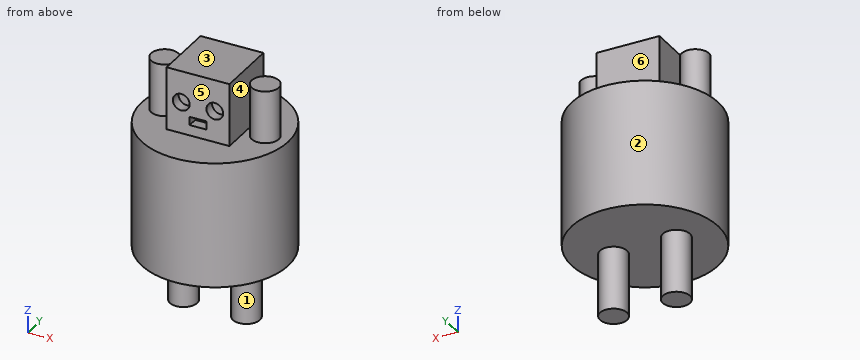
```python
from build123d import *

# Parameters (mm, degrees)
F0_W     = 30
F0_H     = 30
F1_DEPTH = 15
F2_R     = 35
F3_DEPTH = 60
F4_R     = 6.5
F5_DEPTH = 30
F6_R     = 4
F6_W     = 8
F6_H     = 4
F7_DEPTH = 5
F8_R     = 6.5
F9_DEPTH = 25


with BuildPart() as f1:
    # F0 (on Front) → F1 (new body, symmetric)
    with BuildSketch(Plane.XZ):
        with Locations((0, 40)):
            Rectangle(F0_W, F0_H)
    extrude(amount=F1_DEPTH, both=True)

    # F2 (on face) → F3 (join)
    with BuildSketch(Plane(origin=(0, 0, 25), x_dir=(1, 0, 0), z_dir=(0, 0, -1))):
        Circle(F2_R)
    extrude(amount=F3_DEPTH)

    # F4 (on face) → F5 (join)
    with BuildSketch(Plane(origin=(0, 0, -35), x_dir=(1, 0, 0), z_dir=(0, 0, -1))):
        with Locations((-15, 0)):
            Circle(F4_R)
        with Locations((15, 0)):
            Circle(F4_R)
    extrude(amount=F5_DEPTH)

    # F6 (on face) → F7 (cut)
    with BuildSketch(Plane.XZ.offset(15)):
        with Locations((-8, 40)):
            Circle(F6_R)
        with Locations((8, 40)):
            Circle(F6_R)
        with Locations((0, 32)):
            Rectangle(F6_W, F6_H)
    extrude(amount=-F7_DEPTH, mode=Mode.SUBTRACT)

    # F8 (on face) → F9 (join)
    with BuildSketch(Plane.XY.offset(25)):
        with Locations((-24, 0)):
            Circle(F8_R)
        with Locations((24, 0)):
            Circle(F8_R)
    extrude(amount=F9_DEPTH)


solid = f1.part
```
Check sheet for the modelled part. Datum: model origin and axes. Units: mm. Face numbers are marked on the shaded views. A direction names the side the tool comes from. Round coordinates to 2 decimals unless told otherwise and drop trailing zeros. Order: outer loops, then holes, each group sorted by start corner. A loop starts at its lowest first (then second) coordinate and runs counter-clockwise, first axis right, second up. Notation, with made-up numbers: (-38, -28) -> (-32, -28) arc R23 cw to (-32, -14) -> close; hole circle Ø10 at (45, -30.75). An arc over 180 degrees is marked (long way). One line per item, written item: value. Start each with the question number.
Q1. Cross-section at A-A (z = 40). Record the boundary of the cut face in (x, y), and give its area (3 significant figures).
Q2. Cross-section at B-B (x = 0). Record the boundary of the cut face in (y, z).
Q3. Gauge pin test, flat ends, axial feed: pin 1 Ø2 at (y, z) = (-13.5, 32) entering from -X; pin 2 Ø10.5 at (x, z) = (8, 40) entering from +Y; pin 3 Ø24 at (x, z) = (-3, 46.5) entering from -Y; pin 4 Ø21 at (x, y) = (9, -4.5) entering from -Z. Record the tip position at first contact, or that the pin passes through.
Q4. Set-up check for the marked faces 4, 5 and 6: record each of +Z, -Z, +X, -X, +Y, -Y from which the full face is reachable in a straight line by a thin tool's end or side.
Q5. Cross-section at C-C (z = -48). Record the boundary of the cut face in (x, y), and give its area (3 significant figures).
Q6. Mould release check, pull along X, two halves, no side actions. Record for the marked faces 1, 2 and 3: pulls with the +X half, pulls with the -X half, needs draft (parallel to the pull), parting line crosses it, or undercut.
Q7. Thickness scan on line 1 (Z direction, x = 8, y = -11.55); line 2 (X direction, y = 6, z = 25.5); line 3 (Z direction, x = 18, y = 20). Record the ranges inside material, lowest first.
Q8. Cross-section at D-D (y = 0). Record the boundary of the cut face in (x, z), and give its area (3 significant figures).
Completed:
1. outline: circle Ø13 at (-24, 0); (-15, -15) -> (-12, -15) -> (-12, -10) -> (-4, -10) -> (-4, -15) -> (4, -15) -> (4, -10) -> (12, -10) -> (12, -15) -> (15, -15) -> (15, 15) -> (-15, 15) -> close; circle Ø13 at (24, 0)
1. area: 1,090 mm²
2. outline: (-35, -35) -> (35, -35) -> (35, 25) -> (15, 25) -> (15, 55) -> (-15, 55) -> (-15, 34) -> (-10, 34) -> (-10, 30) -> (-15, 30) -> (-15, 25) -> (-35, 25) -> close
3. pin 1: stops at x = -15
3. pin 2: stops at y = 15
3. pin 3: stops at y = -15
3. pin 4: stops at z = -65
4. face 4: +Z, +Y, -Y
4. face 5: +Z, +X, -X, -Y
4. face 6: +Z, +X, -X, +Y
5. outline: circle Ø13 at (-15, 0); circle Ø13 at (15, 0)
5. area: 265 mm²
6. face 1: undercut
6. face 2: parting line crosses it
6. face 3: needs draft
7. line 1: z = -35 to 36, 44 to 55
7. line 2: x = -26.5 to -21.5, -15 to 15, 21.5 to 26.5
7. line 3: z = -35 to 25
8. outline: (-35, -35) -> (-21.5, -35) -> (-21.5, -65) -> (-8.5, -65) -> (-8.5, -35) -> (8.5, -35) -> (8.5, -65) -> (21.5, -65) -> (21.5, -35) -> (35, -35) -> (35, 25) -> (30.5, 25) -> (30.5, 50) -> (17.5, 50) -> (17.5, 25) -> (15, 25) -> (15, 55) -> (-15, 55) -> (-15, 25) -> (-17.5, 25) -> (-17.5, 50) -> (-30.5, 50) -> (-30.5, 25) -> (-35, 25) -> close
8. area: 6,530 mm²
